Part model, mm, in its own coordinate system. A direction names the side the tool comes from. Give positions to 0.01 mm unless a question says otherwise; leave off trailing zeros. Order: outer loops, then holes, each group sorted by start corner. A loop starts at its lowest first (then second) coordinate and runs counter-clockwise, first axis right, second up. Notation, with made-up numbers: (36, 36.25) - (60, 36.25) arc R18 ccw to (60, 41.25) - close; hole circle Ø1 at (52, 12.25). An arc over 180 degrees is marked (long way). One line per item, written item: value.
```python
from build123d import *

# Parameters (mm, degrees)
SKETCH_1_R      = 2.55
EXTRUDE_1_DEPTH = 200
FILLET_1_R      = 1


with BuildPart() as part:
    # 草图1 → 凸台-拉伸1 (new body)
    with BuildSketch(Plane.XY):
        Polygon((4.62194142, 1.905266374), (6.694733626, 3.97805858), (6.694733626, 6.205266374), (5.094733626, 6.205266374), (5.094733626, 8.005266374), (11.994733626, 8.005266374), (11.994733626, 1.105266374), (10.194733626, 1.105266374), (10.194733626, 2.705266374), (7.967525833, 2.705266374), (5.894733626, 0.632474167), (5.894733626, -4.62194142), (7.967525833, -6.694733626), (10.194733626, -6.694733626), (10.194733626, -5.094733626), (11.994733626, -5.094733626), (11.994733626, -11.994733626), (5.094733626, -11.994733626), (5.094733626, -10.194733626), (6.694733626, -10.194733626), (6.694733626, -7.967525833), (4.62194142, -5.894733626), (-0.632474167, -5.894733626), (-2.705266374, -7.967525833), (-2.705266374, -10.194733626), (-1.105266374, -10.194733626), (-1.105266374, -11.994733626), (-8.005266374, -11.994733626), (-8.005266374, -5.094733626), (-6.205266374, -5.094733626), (-6.205266374, -6.694733626), (-3.97805858, -6.694733626), (-1.905266374, -4.62194142), (-1.905266374, 0.632474167), (-3.97805858, 2.705266374), (-6.205266374, 2.705266374), (-6.205266374, 1.105266374), (-8.005266374, 1.105266374), (-8.005266374, 8.005266374), (-1.105266374, 8.005266374), (-1.105266374, 6.205266374), (-2.705266374, 6.205266374), (-2.705266374, 3.97805858), (-0.632474167, 1.905266374), align=None)
        with Locations((1.994733626, -1.994733626)):
            Circle(SKETCH_1_R, mode=Mode.SUBTRACT)
    extrude(amount=EXTRUDE_1_DEPTH)

    # 圆角1
    fillet_1_edges = [part.edges().sort_by_distance(p)[0] for p in [
        (-8.005266374, -11.994733626, 100),
        (-8.005266374, 8.005266374, 100),
        (11.994733626, 8.005266374, 100),
        (11.994733626, -11.994733626, 100),
    ]]
    fillet(fillet_1_edges, radius=FILLET_1_R)


solid = part.part
```
1) Slice it at A-A on x = 2.25. Write the cut outline in (y, z).
Answer:
outline: (-5.89, 0) - (-4.53, 0) - (-4.53, 200) - (-5.89, 200) - close; (0.54, 0) - (1.91, 0) - (1.91, 200) - (0.54, 200) - close
2) Wall check: line 1 along X through (y, z) = (6.75, 62); line 2 along X through (y, z) = (1.25, 22); line 3 along Y through (x, z) = (-5.5, 122). Give the ranges that are in metal, low to high. Write a range as [from, to].
Answer:
line 1: x = [-8.01, -1.11], [5.09, 11.99]
line 2: x = [-8.01, -6.21], [-2.52, 6.51], [10.19, 11.99]
line 3: y = [-11.99, -6.69], [2.71, 8.01]
3) Two-plate mould, pull along X, no slides. Class faces 1 (the face through (-0.553, -1.883, 98.6)), 2 (the face through (4, 0, 200)), 3 (the face through (11.995, 4, 99)): pulls with the +X half, pulls with the -X half, needs draft (parallel to the pull), parting line crosses it, or undercut.
Answer:
face 1: undercut
face 2: needs draft
face 3: pulls with the +X half
4) Which spindle directions (+Z, -Z, +X, -X, +Y, -Y) get a long thin tool onto all of the face, cutting with end or side? Do faces 4 (the face through (-1.905, -2, 99)), 5 (the face through (2, -5.895, 99)), 6 (the face through (2, 1.905, 99)). Say none if no direction does.
Answer:
face 4: +Z, -Z, -X
face 5: +Z, -Z, -Y
face 6: +Z, -Z, +Y
5) Drop flat-ended pins along their axis: P1, Ø5, axis at x = -4.5, y = -3.5, coming from the -Z side; P2, Ø4, axis at y = -2.5, z = 120.5, coming from the +X side; P3, Ø0.5, axis at y = -11.5, z = 74, coming from the -X side; P4, Ø2, axis at x = 3.5, z = 28, coming from the -Y side. Give the stop position or say it passes through.
Answer:
P1: stops at z = 0
P2: stops at x = 5.89
P3: stops at x = -7.97
P4: stops at y = -5.89
